from build123d import *

# Parameters (mm, degrees)
SKETCH1_R           = 30
BOSS_EXTRUDE1_DEPTH = 36
FILLET1_R           = 22
FILLET2_R           = 22
SKETCH3_OUTSIDE_W   = 84.256
SKETCH3_OUTSIDE_H   = 84.256
SKETCH3_OUTSIDE_R   = 24
CUT_EXTRUDE2_DEPTH  = 14
CUT_EXTRUDE3_DEPTH  = 16
SKETCH6_W           = 34.957116586
SKETCH6_H           = 10.5
CUT_EXTRUDE9_DEPTH  = 12


with BuildPart() as part:
    # Sketch1 → Boss-Extrude1 (new, symmetric)
    with BuildSketch(Plane(origin=(0, 0, 0), x_dir=(1, 0, 0), z_dir=(0, 1, 0))):
        with Locations(Location((0, 0, 0), (0, 0, 270))):
            Circle(SKETCH1_R)
    extrude(amount=BOSS_EXTRUDE1_DEPTH, both=True)

    # Fillet1
    fillet1_edges = [part.edges().sort_by_distance(p)[0] for p in [
        (0, 36, -30),
    ]]
    fillet(fillet1_edges, radius=FILLET1_R)

    # Fillet2
    fillet2_edges = [part.edges().sort_by_distance(p)[0] for p in [
        (0, -36, -30),
    ]]
    fillet(fillet2_edges, radius=FILLET2_R)

    # Sketch3 outside → Cut-Extrude2 (cut, symmetric)
    with BuildSketch(Plane(origin=(0, 0, 0), x_dir=(1, 0, 0), z_dir=(0, 1, 0))):
        Rectangle(SKETCH3_OUTSIDE_W, SKETCH3_OUTSIDE_H)
        with Locations(Location((0, 0, 0), (0, 0, 270))):
            Circle(SKETCH3_OUTSIDE_R, mode=Mode.SUBTRACT)
    extrude(amount=CUT_EXTRUDE2_DEPTH, both=True, mode=Mode.SUBTRACT)

    # Sketch4 → Cut-Extrude3 (cut)
    with BuildSketch(Plane(origin=(0, 36, 0), x_dir=(1, 0, 0), z_dir=(0, 1, 0))):
        with BuildLine():
            ThreePointArc((6.036348234, 5.25), (0, 8), (-6.036348234, 5.25))
            Line((-6.036348234, 5.25), (6.036348234, 5.25))
        make_face()
        with BuildLine():
            ThreePointArc((17.478558293, 5.25), (0, 18.25), (-17.478558293, 5.25))
            Line((-17.478558293, 5.25), (-6.036348234, 5.25))
            ThreePointArc((-6.036348234, 5.25), (0, 8), (6.036348234, 5.25))
            Line((6.036348234, 5.25), (17.478558293, 5.25))
        make_face()
        with BuildLine():
            Line((6.036348234, -5.25), (-6.036348234, -5.25))
            ThreePointArc((-6.036348234, -5.25), (0, -8), (6.036348234, -5.25))
        make_face()
        with BuildLine():
            Line((-6.036348234, -5.25), (-17.478558293, -5.25))
            ThreePointArc((-17.478558293, -5.25), (0, -18.25), (17.478558293, -5.25))
            Line((17.478558293, -5.25), (6.036348234, -5.25))
            ThreePointArc((6.036348234, -5.25), (0, -8), (-6.036348234, -5.25))
        make_face()
    extrude(amount=-CUT_EXTRUDE3_DEPTH, mode=Mode.SUBTRACT)

    # Sketch6 → Cut-Extrude9 (cut)
    with BuildSketch(Plane(origin=(0, 20, 0), x_dir=(1, 0, 0), z_dir=(0, 1, 0))):
        Rectangle(SKETCH6_W, SKETCH6_H)
    extrude(amount=CUT_EXTRUDE9_DEPTH, mode=Mode.SUBTRACT)


solid = part.part
Geometry: final body of the model. Coordinates: model frame, mm. A direction names the side the tool comes from. Coordinates: 2 decimals unless noted, no trailing zeros. Order: outer loops, then holes, each group sorted by start corner. A loop starts at its lowest first (then second) coordinate and runs counter-clockwise, first axis right, second up.
1) Section A-A (y = -1). Return loops of the section in (x, z).
Result sheet:
outline: circle Ø48 at (0, 0)
2) Draft query along X for faces 3 (the flat face through (-13.5, 14, -20.1)), 4 (the cylindrical face through (7.21, -0.2, 22.89)), 5 (the flat face through (0, 20, 0)). Return one class per face: released by +X, released by -X, zero draft, split by the parting line, or undercut.
Result sheet:
face 3: zero draft
face 4: split by the parting line
face 5: undercut
3) First-contact query: P1, Ø3, axis at y = 29, z = -2.5, coming from the -X side; P2, Ø6, axis at y = -28, z = 2.5, coming from the -X side; P3, Ø6, axis at x = -6.5, y = -5.5, coming from the +Z side. Flat tips, straight axial feed; report the tip coordinate or a pass-through.
Result sheet:
P1: stops at x = -25.26
P2: stops at x = -26.96
P3: stops at z = 23.74
4) Set-up query: faces 1 (the flat face through (0, 36, 0)), 2 (the flat face through (17.479, 26, 0)). Return all of +Z, -Z, +X, -X, +Y, -Y with unobstructed straight access to the full face (end or side cutting, diameter ignored); none if empty.
Result sheet:
face 1: +Z, -Z, +X, -X, +Y
face 2: none
5) Ray query, probe 1 along Y at (x, z) = (3.5, 1.5); probe 2 along Y at (x, z) = (26, 9); probe 3 along Y at (x, z) = (-6, 6). Return the intervals inside material, ascending.
Result sheet:
probe 1: y = -36 to 20, 32 to 36
probe 2: y = -24.16 to -14, 14 to 24.16
probe 3: y = -35.99 to 20
